The listing builds one solid part. Answer for the finished solid, in the listing's coordinates (mm). A direction names the side the tool comes from. Coordinates: 2 decimals unless noted, no trailing zeros. Write each loop counter-clockwise with the first axis right and the second up, starting at its lowest first coordinate (ties: lowest second). Pieces come first, ordered by that corner, then holes. Notation, with made-up numbers: M 18.5,20 L 30.5,20 A5 cw 30.5,24 Z; hole C 10.25,-9.75 d9. An arc over 180 degrees is marked long. Answer as CSV lines item,"result".
```python
from build123d import *

# Parameters (mm, degrees)
F1_DEPTH = 25.4
F2_R     = 10.634514
F3_DEPTH = 25.4
F4_R     = 5.192433
F5_DEPTH = 50.8


with BuildPart() as f1:
    # F0 (on Top) → F1 (new body)
    with BuildSketch(Plane.XY):
        Polygon((-0.495151, 44.171312), (-38.005903, -22.514469), (38.501054, -21.656843), align=None)
    extrude(amount=F1_DEPTH)

    # F2 (on face) → F3 (join)
    with BuildSketch(Plane.XY.offset(25.4)):
        Circle(F2_R)
    extrude(amount=F3_DEPTH)

    # F4 (on face) → F5 (join)
    with BuildSketch(Plane.XY.offset(50.8)):
        Circle(F4_R)
    extrude(amount=-F5_DEPTH)


solid = f1.part
```
Q1. Find section D-D (z = 15). Give the vertices of the cut face in (x, y).
Output:
outline,"M -38.01,-22.51 L 38.5,-21.66 L -0.5,44.17 Z"
Q2. Find section B-B (x = -4.5). Give the vertices of the cut face in (y, z), and give its area (3 significant figures).
Output:
outline,"M -22.14,0 L 37.05,0 L 37.05,25.4 L 9.64,25.4 L 9.64,50.8 L -9.64,50.8 L -9.64,25.4 L -22.14,25.4 Z"
area,"1,990 mm2"
Q3. For faces 1 (the cylindrical face through (-2.31, -10.38, 37.92)), 2 (the flat face through (-18.988, 11.295, 12.522)), determine the directions among +Z, -Z, +X, -X, +Y, -Y from which every point of the face is accessible in a straight line to the end or side of a thin tool.
Output:
face 1,"+Z"
face 2,"+Z, -Z, -X, +Y"
Q4. Straight lines are drawn through the part: line 1 (X direction, y = 0.5, z = 31); line 2 (Z direction, x = -23.5, y = -3.5); line 3 (Y direction, x = -23, z = 7.5). For each, find the intervals that lie inside material, in ascending order.
Output:
line 1,"-10.62 to 10.62"
line 2,"0 to 25.4"
line 3,"-22.35 to 4.16"
Q5. Find section A-A (y = 6). Give the vertices of the cut face in (x, z).
Output:
outline,"M -21.97,0 L 22.12,0 L 22.12,25.4 L 8.78,25.4 L 8.78,50.8 L -8.78,50.8 L -8.78,25.4 L -21.97,25.4 Z"
Q6. Find section C-C (z = 35). Give the vertices of the cut face in (x, y), and give its area (3 significant figures).
Output:
outline,"C 0,0 d21.27"
area,"355 mm2"
Q7. Flat-ended cylindrical pins translate along their axes: pin 1 Ø3 at (x, y) = (13.5, -5.5) entering from +Z; pin 2 Ø2 at (x, z) = (6.5, 40) entering from +Y; pin 3 Ø1 at (x, z) = (-8.5, 21) entering from +Y. Find the tip coordinate at first contact, or state that the pin passes through.
Output:
pin 1,"z = 25.4"
pin 2,"y = 9.1"
pin 3,"y = 30.83"
